Here's how the part is built. I have some questions about the finished solid (model axes, mm). A direction names the side the tool comes from. Give positions to 0.01 mm unless a question says otherwise; leave off trailing zeros. Write each loop counter-clockwise with the first axis right and the second up, starting at its lowest first coordinate (ties: lowest second). Pieces come first, ordered by that corner, then holes. Notation, with made-up numbers: M -4,47 L 12,47 A19 ccw 12,78 Z; hole C -2,47.5 d6. An arc over 180 degrees is marked long. Answer as CSV lines item,"result". Start each with the question number.
Q1. For pin 1 (1 mm diameter, centred on y = -0.5, z = -1, fed in from +X), with a flat end and sliding along its axis, tell me the tip position at first contact or that it passes through.
Q2. Thinking about a two-plate mould opening in Z: for faces 1 (the flat face through (8, -1.6, 0)), 2 (the flat face through (-13, 0, 2)), 3 (the flat face through (-0.2, 1.1, 3)), 4 (the flat face through (-0.2, -1.1, -2)), which applies, +Z half, -Z half, draft (parallel to the pull), parting line (faces both ways), or undercut?
Q3. Suppose I cut it at A-A (y = 0). Write out the boundary of the cut face in (x, z).
Q4. If I drill on line 1 along Z through (x, y) = (-7.75, 0.25); line 2 along X through (y, z) = (0, 1.25); line 3 along Y through (x, z) = (-3.5, -1.15), over which ranges is the centre line in solid material (lowest first)?
Q5. Suppose I cut it at D-D (x = -5.25). Write out the boundary of the cut face in (y, z), then the cut area to 3 significant figures.
Q6. Suppose I cut it at C-C (x = 0). Write out the boundary of the cut face in (y, z), then the cut area to 3 significant figures.
Q7. Suppose I cut it at B-B (z = 0). Write out the boundary of the cut face in (x, y), then the cut area to 3 significant figures.
Q8. On a 3-axis mill with a long thin cutter (end or side, diameter ignored), from which of +Z, -Z, +X, -X, +Y, -Y can I reach the whole of each face in a straight line? I mean faces 5 (the flat face through (-8, 0, -1.6)), 6 (the flat face through (8, 1.6, 0)), 7 (the cylindrical face through (0.27, -0.86, 0.54)). Say none if no direction works.
```python
from build123d import *

# Parameters (mm, degrees)
SKETCH3_R             = 3
BOSS_EXTRUDE1_DEPTH   = 6
BOSS_EXTRUDE2_START   = -3
SKETCH4_W             = 6
SKETCH4_H             = 6
BOSS_EXTRUDE2_DEPTH   = 13
SKETCH5_W             = 3.2
SKETCH5_H             = 3.2
CUT_EXTRUDE1_DEPTH    = 10
SKETCH6_R             = 0.9
CUT_EXTRUDE2_DEPTH    = 15.628738838
MIRROR2_DEPTH         = 6
MIRROR2_2_OUTLINE_W   = 10
MIRROR2_2_OUTLINE_H   = 3.2
MIRROR2_2_DEPTH       = 1.4
MIRROR2_START         = 4.6
MIRROR2_3_OUTLINE_W   = 10
MIRROR2_3_OUTLINE_H   = 3.2
MIRROR2_3_DEPTH       = 1.4
SKETCH8_W             = 26
SKETCH8_H             = 6
CUT_EXTRUDE3_DEPTH    = 1
FILLET1_R             = 0.5
BODY_MOVE_COPY1_ANGLE = 90


with BuildPart() as part:
    # Sketch3 → Boss-Extrude1 (new body)
    with BuildSketch(Plane(origin=(0, 0, 0), x_dir=(1, 0, 0), z_dir=(0, 1, 0))):
        with Locations(Location((0, 0, 0), (0, 0, 270))):
            Circle(SKETCH3_R)
    extrude(amount=BOSS_EXTRUDE1_DEPTH)

    # Sketch4 → Boss-Extrude2 (add)
    with BuildSketch(Plane.ZY.offset(3).offset(BOSS_EXTRUDE2_START)):
        with Locations((0, 3)):
            Rectangle(SKETCH4_W, SKETCH4_H)
    extrude(amount=BOSS_EXTRUDE2_DEPTH)

    # Sketch5 → Cut-Extrude1 (cut)
    with BuildSketch(Plane.ZY.offset(13)):
        with Locations((0, 3)):
            Rectangle(SKETCH5_W, SKETCH5_H)
    extrude(amount=-CUT_EXTRUDE1_DEPTH, mode=Mode.SUBTRACT)

    # Sketch6 → Cut-Extrude2 (cut, through all)
    with BuildSketch(Plane(origin=(0, 6, 0), x_dir=(1, 0, 0), z_dir=(0, 1, 0))):
        with Locations(Location((0, 0, 0), (0, 0, 270))):
            Circle(SKETCH6_R)
    extrude(amount=-CUT_EXTRUDE2_DEPTH, mode=Mode.SUBTRACT)

    # Mirror2: read off the stored shape, not the designer's step
    # Mirror2 outline → Mirror2 (add)
    with BuildSketch(Plane(origin=(0, 0, 0), x_dir=(1, 0, 0), z_dir=(0, 1, 0))):
        with BuildLine():
            Line((13, 1.6), (13, 3))
            Line((13, 3), (0, 3))
            ThreePointArc((0, 3), (2.121320344, 2.121320344), (3, 0))
            Line((3, 0), (3, 1.6))
            Line((3, 1.6), (13, 1.6))
        make_face()
        with BuildLine():
            Line((13, -3), (13, -1.6))
            Line((13, -1.6), (3, -1.6))
            Line((3, -1.6), (3, 0))
            ThreePointArc((3, 0), (2.121320344, -2.121320344), (0, -3))
            Line((0, -3), (13, -3))
        make_face()
    extrude(amount=MIRROR2_DEPTH)

    # Mirror2 2 outline → Mirror2 2 (add)
    with BuildSketch(Plane(origin=(0, 0, 0), x_dir=(1, 0, 0), z_dir=(0, 1, 0))):
        with Locations((8, 0)):
            Rectangle(MIRROR2_2_OUTLINE_W, MIRROR2_2_OUTLINE_H)
    extrude(amount=MIRROR2_2_DEPTH)

    # Mirror2 3 outline → Mirror2 3 (add)
    with BuildSketch(Plane(origin=(0, 0, 0), x_dir=(1, 0, 0), z_dir=(0, 1, 0)).offset(MIRROR2_START)):
        with Locations((8, 0)):
            Rectangle(MIRROR2_3_OUTLINE_W, MIRROR2_3_OUTLINE_H)
    extrude(amount=MIRROR2_3_DEPTH)

    # Sketch8 → Cut-Extrude3 (cut)
    with BuildSketch(Plane.XZ):
        Rectangle(SKETCH8_W, SKETCH8_H)
    extrude(amount=-CUT_EXTRUDE3_DEPTH, mode=Mode.SUBTRACT)

    # Fillet1
    fillet1_edges = [part.edges().sort_by_distance(p)[0] for p in [
        (0, 1, 3),
        (0, 1, -3),
        (0, 6, 3),
        (0, 6, -3),
    ]]
    fillet(fillet1_edges, radius=FILLET1_R)


with BuildPart() as part_1:
    # Body-Move/Copy1: moved
    add(part.part.rotate(Axis((0, 3.5, 0), (1, 0, 0)), BODY_MOVE_COPY1_ANGLE))


with BuildPart() as part_2:
    # Body-Move/Copy2: read off the stored shape, not the designer's step
    # Body-Move/Copy2: moved
    add(part_1.part.moved(Location((0, -3.5, 0.5))))


solid = part_2.part
```
Resolved:
1,pin 1,"x = 3"
2,face 1,"undercut"
2,face 2,"draft"
2,face 3,"+Z half"
2,face 4,"-Z half"
3,outline,"M -13,-2 L -0.9,-2 L -0.9,3 L -13,3 L -13,1.6 L -3,1.6 L -3,-1.6 L -13,-1.6 Z; M 0.9,-2 L 13,-2 L 13,-1.6 L 3,-1.6 L 3,1.6 L 13,1.6 L 13,3 L 0.9,3 Z"
4,line 1,"-2 to -1.6, 1.6 to 3"
4,line 2,"-3 to -0.9, 0.9 to 3"
4,line 3,"-3 to -1.6, 1.6 to 3"
5,outline,"M -3,-1.5 A0.5 ccw -2.5,-2 L 2.5,-2 A0.5 ccw 3,-1.5 L 3,2.5 A0.5 ccw 2.5,3 L -2.5,3 A0.5 ccw -3,2.5 Z; hole M -1.6,-1.6 L 1.6,-1.6 L 1.6,1.6 L -1.6,1.6 Z"
5,area,"19.5 mm^2"
6,outline,"M -3,-1.5 A0.5 ccw -2.5,-2 L -0.9,-2 L -0.9,3 L -2.5,3 A0.5 ccw -3,2.5 Z; M 0.9,-2 L 2.5,-2 A0.5 ccw 3,-1.5 L 3,2.5 A0.5 ccw 2.5,3 L 0.9,3 Z"
6,area,"20.8 mm^2"
7,outline,"M -13,-3 L 13,-3 L 13,-1.6 L 3,-1.6 L 3,1.6 L 13,1.6 L 13,3 L -13,3 L -13,1.6 L -3,1.6 L -3,-1.6 L -13,-1.6 Z; hole C 0,0 d1.8"
7,area,"89.5 mm^2"
8,face 5,"-X"
8,face 6,"+X"
8,face 7,"+Z, -Z"
